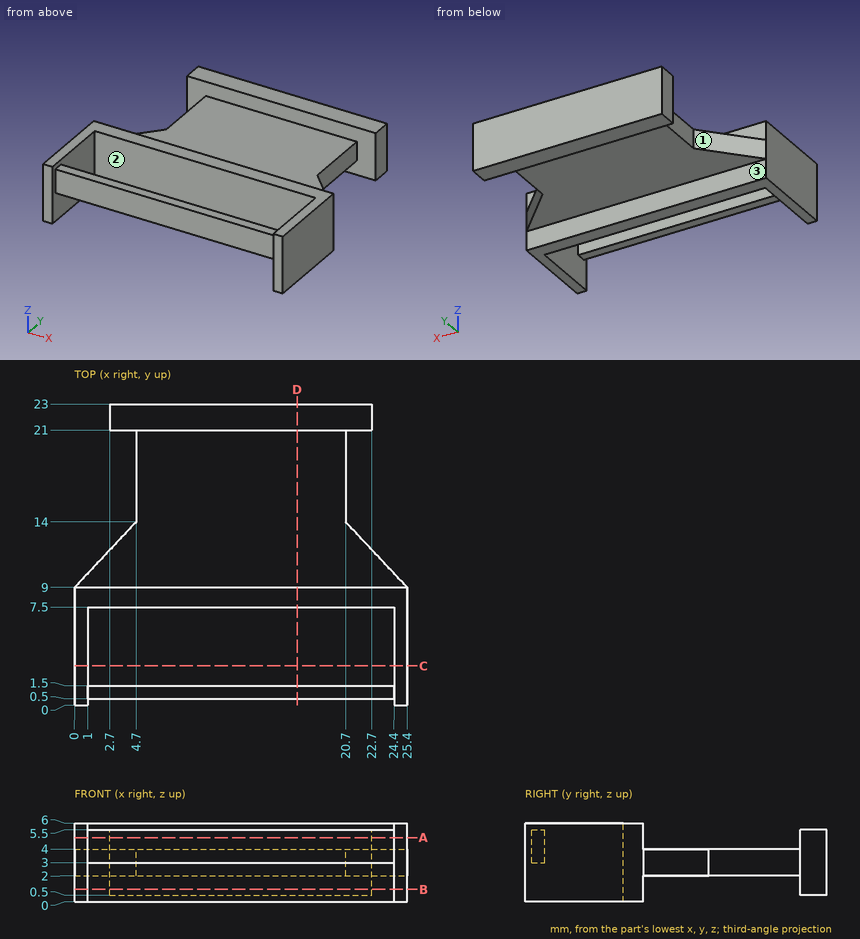
Study the drawing (mm; zero at the part's minimum x, y, z) and answer. A direction names the side the tool comes from. Give positions to 0.01 mm unless a question says otherwise; leave off trailing zeros. Order: outer loops, then holes, each group sorted by start corner. A loop starts at its lowest first (then second) coordinate and runs counter-clockwise, first axis right, second up. Notation, with made-up numbers: (54.5, 12.25) - (73.5, 12.25) arc R23 cw to (73.5, 48.25) - close; hole circle Ø3 at (-15, 19.5). An arc over 180 degrees is marked (long way). Answer as CSV lines item,"result". Start each with the question number.
Q1. The part is cut by section B-B (z = 0.95). Write down the section's boundary in (x, y).
Q2. The part is cut by section D-D (x = 17). Write down the section's boundary in (y, z).
Q3. The part is cut by section A-A (z = 4.9). Write down the section's boundary in (x, y).
Q4. For the marked faces 1, 2 and 3, determine the directions among +Z, -Z, +X, -X, +Y, -Y from which every point of the face is accessible in a straight line to the end or side of a thin tool.
Q5. Given pin 1 Ø0.6 at (y, z) = (18.5, 3) entering from -X; pin 2 Ø3 at (x, y) = (6, 12) entering from -Z; pin 3 Ø1 at (x, y) = (14.5, 22) entering from +Z, each flat-ended and moving along its own axis, determine where each tip first touches the part or whether it passes through.
Q6. The part is cut by section C-C (y = 3). Write down the section's boundary in (x, z).
Q7. Find the intervals of material crossed by L1, parallel to Y at x = 9, z = 4.15; L2, parallel to X at y = 5.75, z = 1.8; L3, parallel to Y at x = 21.75, z = 1.6, in increasing order. Write a range as [from, to].
Check result:
1,outline,"(0, 0) - (1, 0) - (1, 7.5) - (24.4, 7.5) - (24.4, 0) - (25.4, 0) - (25.4, 9) - (0, 9) - close; (2.7, 21) - (22.7, 21) - (22.7, 23) - (2.7, 23) - close"
2,outline,"(0.5, 3) - (1.5, 3) - (1.5, 5.5) - (0.5, 5.5) - close; (7.5, 0) - (9, 0) - (9, 2) - (21, 2) - (21, 0.5) - (23, 0.5) - (23, 5.5) - (21, 5.5) - (21, 4) - (9, 4) - (9, 6) - (7.5, 6) - close"
3,outline,"(0, 0) - (1, 0) - (1, 0.5) - (24.4, 0.5) - (24.4, 0) - (25.4, 0) - (25.4, 9) - (0, 9) - close; (2.7, 21) - (22.7, 21) - (22.7, 23) - (2.7, 23) - close; hole (1, 1.5) - (24.4, 1.5) - (24.4, 7.5) - (1, 7.5) - close"
4,face 1,"+Z, -Z, -X"
4,face 2,"+Z, -Z"
4,face 3,"-Z, +X, -X"
5,pin 1,"stops at x = 4.7"
5,pin 2,"stops at z = 2"
5,pin 3,"stops at z = 5.5"
6,outline,"(0, 0) - (1, 0) - (1, 6) - (0, 6) - close; (24.4, 0) - (25.4, 0) - (25.4, 6) - (24.4, 6) - close"
7,L1,"y = [0.5, 1.5], [7.5, 9], [21, 23]"
7,L2,"x = [0, 1], [24.4, 25.4]"
7,L3,"y = [7.5, 9], [21, 23]"
